Input: dimensioned drawing with shaded views. Units: mm. Origin: part minimum x, y, z. Coordinates: 2 decimals unless noted, no trailing zeros. Write each loop counter-clockwise with the first axis right and the second up, starting at its lowest first coordinate (ties: lowest second). Pieces come first, ordered by that corner, then holes. Notation, with made-up numbers: M -27.75,65 L -6.75,65 A17 cw -6.75,83 Z; hole C -26.75,10 d6. An arc over 180 degrees is marked long. Write each question's results on one line, items separated by ' | '. Start each with the question number.
1. Section query D-D, the plane x = 47.5. Output: boundary loops of the cut face in (y, z).
2. First-contact query: pin 1 (1 mm diameter, centred on x = 23.5, z = 2, fed in from -Y); pin 2 (0.8 mm diameter, centred on x = 7.5, y = 24.5, fed in from +Z). Flat tips, straight axial feed; report the tip coordinate or a pass-through.
3. Section query B-B, the plane y = 38. Output: boundary loops of the cut face in (x, z), and give its area (3 significant figures).
4. Section query A-A, the plane x = 68.6. Output: boundary loops of the cut face in (y, z).
5. Ray query, probe 1 along X at (y, z) = (31.5, 3.7); probe 2 along Y at (x, z) = (4, 1.4); probe 3 along X at (y, z) = (37, 1). Return the intervals inside material, ascending.
6. Section query C-C, the plane z = 2.15. Output: boundary loops of the cut face in (x, y).
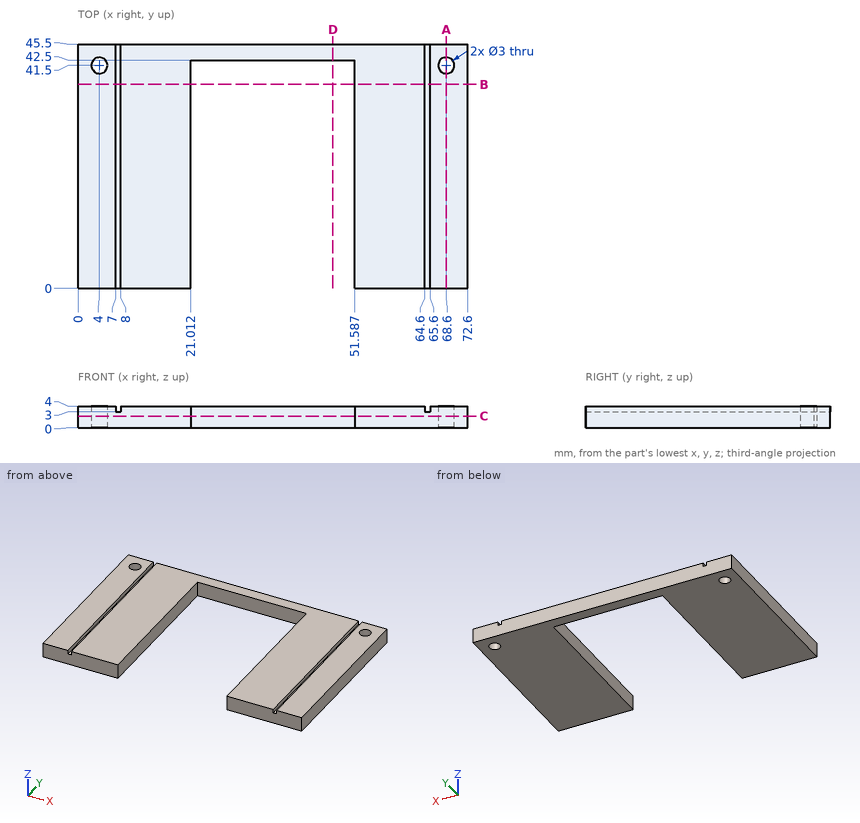
Answer:
1) outline: M 42.5,0 L 45.5,0 L 45.5,4 L 42.5,4 Z
2) pin 1: y = 42.5 | pin 2: z = 3
3) outline: M 0,0 L 21.01,0 L 21.01,4 L 8,4 L 8,3 L 7,3 L 7,4 L 0,4 Z; M 51.59,0 L 72.6,0 L 72.6,4 L 65.6,4 L 65.6,3 L 64.6,3 L 64.6,4 L 51.59,4 Z | area: 166 mm^2
4) outline: M 0,0 L 40,0 L 40,4 L 0,4 Z; M 43,0 L 45.5,0 L 45.5,4 L 43,4 Z
5) probe 1: 0 to 7, 8 to 21.01, 51.59 to 64.6, 65.6 to 72.6 | probe 2: 0 to 40, 43 to 45.5 | probe 3: 0 to 21.01, 51.59 to 72.6
6) outline: M 0,0 L 21.01,0 L 21.01,42.5 L 51.59,42.5 L 51.59,0 L 72.6,0 L 72.6,45.5 L 0,45.5 Z; hole C 4,41.5 d3; hole C 68.6,41.5 d3
